```python
from build123d import *

# Parameters (mm, degrees)
EXTRUDE_1_DEPTH     = 50
SKETCH_2_R          = 1.6
CUT_EXTRUDE_1_DEPTH = 4
SKETCH_3_R          = 1.6
CUT_EXTRUDE_2_DEPTH = 26


with BuildPart() as part:
    # ｽｹｯﾁ1 → ﾎﾞｽ - 押し出し1 (new body)
    with BuildSketch(Plane(origin=(0, 0, 0), x_dir=(0, 0, -1), z_dir=(1, 0, 0))):
        Polygon((0, 50), (25, 50), (25, 47), (3, 47), (3, 0), (0, 0), align=None)
    extrude(amount=EXTRUDE_1_DEPTH)

    # ｽｹｯﾁ2 → ｶｯﾄ - 押し出し1 (cut, through all)
    with BuildSketch(Plane.XZ.offset(-47)):
        with Locations((8.5, -9)):
            Circle(SKETCH_2_R)
        with Locations((8.5, -21)):
            Circle(SKETCH_2_R)
        with Locations((41.5, -9)):
            Circle(SKETCH_2_R)
        with Locations((41.5, -21)):
            Circle(SKETCH_2_R)
    extrude(amount=-CUT_EXTRUDE_1_DEPTH, mode=Mode.SUBTRACT)

    # ｽｹｯﾁ3 → ｶｯﾄ - 押し出し2 (cut, through all)
    with BuildSketch(Plane.XY):
        with Locations((17.5, 7.5)):
            Circle(SKETCH_3_R)
        with Locations((32.5, 7.5)):
            Circle(SKETCH_3_R)
    extrude(amount=-CUT_EXTRUDE_2_DEPTH, mode=Mode.SUBTRACT)


solid = part.part
```
Geometry check sheet. Reference: the model listing, model coordinates, mm. A direction names the side the tool comes from. Coordinates: 2 decimals unless noted, no trailing zeros. Order: outer loops, then holes, each group sorted by start corner. A loop starts at its lowest first (then second) coordinate and runs counter-clockwise, first axis right, second up.
Q1. Sectioned sample at A-A on z = -21. Record the cut outline in (x, y).
Reply:
outline: (0, 47) - (6.9, 47) - (6.9, 50) - (0, 50) - close; (10.1, 47) - (39.9, 47) - (39.9, 50) - (10.1, 50) - close; (43.1, 47) - (50, 47) - (50, 50) - (43.1, 50) - close
Q2. Tool access check on faces 5 (the face through (25, 24, -3)), 6 (the face through (31.23, 6.53, -1.48)). Record the directions out of +Z, -Z, +X, -X, +Y, -Y that give a thin tool (end or side, any length) a straight path to the whole face; none if there is none.
Reply:
face 5: -Z, +X, -X, -Y
face 6: +Z, -Z
Q3. Depth check by flat-ended pin: pin 1 Ø23.5 at (x, y) = (26.5, 15) entering from -Z; pin 2 Ø6.5 at (x, z) = (20.5, -17) entering from -Y; pin 3 Ø3 at (x, z) = (41.5, -9) entering from +Y. Enter the tip coordinate at first touch or a pass-through.
Reply:
pin 1: stops at z = -3
pin 2: stops at y = 47
pin 3: passes through
Q4. Thickness scan on probe 1 along Z at (x, y) = (41.5, 49.05); probe 2 along Y at (x, z) = (32.5, -0.7); probe 3 along Z at (x, y) = (17.5, 30). Record the ranges inside material, lowest first.
Reply:
probe 1: z = -25 to -22.6, -19.4 to -10.6, -7.4 to 0
probe 2: y = 0 to 5.9, 9.1 to 50
probe 3: z = -3 to 0
Q5. Draft check along X on faces 1 (the face through (41.15, 48.48, -10.56)), 2 (the face through (8.292, 48.479, -19.414)), 3 (the face through (0, 34, -2)), 4 (the face through (25, 47, -14)). Enter one of: released by +X, released by -X, zero draft, split by the parting line, or undercut.
Reply:
face 1: undercut
face 2: undercut
face 3: released by -X
face 4: zero draft
Q6. Sectioned sample at C-C on x = 41.5. Record the cut outline in (y, z).
Reply:
outline: (0, -3) - (47, -3) - (47, -7.4) - (50, -7.4) - (50, 0) - (0, 0) - close; (47, -25) - (50, -25) - (50, -22.6) - (47, -22.6) - close; (47, -19.4) - (50, -19.4) - (50, -10.6) - (47, -10.6) - close
Q7. Sectioned sample at D-D on x = 32.5. Record the cut outline in (y, z), and give its area (3 significant figures).
Reply:
outline: (0, -3) - (5.9, -3) - (5.9, 0) - (0, 0) - close; (9.1, -3) - (47, -3) - (47, -25) - (50, -25) - (50, 0) - (9.1, 0) - close
area: 206 mm2
Q8. Sectioned sample at B-B on y = 7.5. Record the cut outline in (x, z).
Reply:
outline: (0, -3) - (15.9, -3) - (15.9, 0) - (0, 0) - close; (19.1, -3) - (30.9, -3) - (30.9, 0) - (19.1, 0) - close; (34.1, -3) - (50, -3) - (50, 0) - (34.1, 0) - close
